```python
from build123d import *

# Parameters (mm, degrees)
F1_DEPTH = 50.8
F2_R     = 25.39999
F4_W     = 61.8233563619
F4_H     = 42.2021473569
F4_W_2   = 44.7444434271
F4_H_2   = 31.3514119965
F5_DEPTH = 50.8


# Not quite as in the source:
# - a fillet or chamfer is up to 0.001 mm smaller than in the source, because OpenCascade refuses the exact size


with BuildPart() as f1:
    # F0 (on Top) → F1 (new body)
    with BuildSketch(Plane.XY):
        with BuildLine():
            Line((-125.9584231198, 326.6096413136), (-125.9584231198, -437.0573322225))
            Line((-125.9584231198, -437.0573322225), (-49.7584231198, -437.0573322225))
            Line((-49.7584231198, -437.0573322225), (77.2415768802, -437.0573322225))
            Line((77.2415768802, -437.0573322225), (77.2415768802, -386.2573322225))
            Line((77.2415768802, -386.2573322225), (-49.7584231198, -386.2573322225))
            Line((-49.7584231198, -386.2573322225), (-49.7584231198, -348.1573322225))
            Line((-49.7584231198, -348.1573322225), (77.2415768802, -348.1573322225))
            Line((77.2415768802, -348.1573322225), (77.2415768802, -297.3573322225))
            Line((77.2415768802, -297.3573322225), (-49.7584231198, -297.3573322225))
            Line((-49.7584231198, -297.3573322225), (-49.7584231198, -259.2573322225))
            Line((-49.7584231198, -259.2573322225), (77.2415768802, -259.2573322225))
            Line((77.2415768802, -259.2573322225), (77.2415768802, -208.4573322225))
            Line((77.2415768802, -208.4573322225), (-49.7584231198, -208.4573322225))
            Line((-49.7584231198, -208.4573322225), (-49.7584231198, 326.6096413136))
            ThreePointArc((-49.7584231198, 326.6096413136), (12.201780711, 376.4463381022), (-23.1943939269, 447.6493859763))
            ThreePointArc((-23.1943939269, 447.6493859763), (-86.3855996742, 517.0444461389), (-149.6523168654, 447.718221991))
            ThreePointArc((-149.6523168654, 447.718221991), (-185.4004633868, 377.8523446501), (-125.9584231198, 326.6096413136))
        make_face()
        with BuildLine():
            ThreePointArc((-86.4201652133, 379.6749489688), (-156.0774751911, 370.9944555466), (-113.7312923812, 426.9792088355))
            ThreePointArc((-113.7312923812, 426.9792088355), (-86.4201652133, 491.6444555466), (-59.1090380455, 426.9792088355))
            ThreePointArc((-59.1090380455, 426.9792088355), (-16.7628552356, 370.9944555466), (-86.4201652133, 379.6749489688))
        make_face(mode=Mode.SUBTRACT)
    extrude(amount=F1_DEPTH)

    # F2 (radius 25.4 in the source; OpenCascade refuses exactly that, so slightly less here)
    f2_edges = [f1.edges().sort_by_distance(p)[0] for p in [
        (-125.958423, -55.223845, 50.8),
        (-49.758423, 59.076155, 50.8),
        (-49.758423, 59.076155, 0),
        (-125.958423, -55.223845, 0),
        (-49.758423, -278.307332, 0),
        (-49.758423, -367.207332, 0),
        (-49.758423, -367.207332, 50.8),
        (-49.758423, -278.307332, 50.8),
    ]]
    fillet(f2_edges, radius=F2_R)

    # F4 (on face) → F5 (cut)
    with BuildSketch(Plane.XY.offset(50.8)):
        with Locations((57.3532550612, -390.556258544)):
            Rectangle(F4_W, F4_H)
        with Locations((74.2137985938, -338.4330382207)):
            Rectangle(F4_W_2, F4_H_2)
    extrude(amount=-F5_DEPTH, mode=Mode.SUBTRACT)


solid = f1.part
```
The model under review builds one solid part; all positions refer to its coordinate system, in mm. A direction names the side the tool comes from. Coordinates: 2 decimals unless noted, no trailing zeros. Write each loop counter-clockwise with the first axis right and the second up, starting at its lowest first coordinate (ties: lowest second). Pieces come first, ordered by that corner, then holes.
1) We need section A-A on x = 1.5. State the section outline as (y, z) points, then the cut area to 3 significant figures.
2) To check wall thickness, follow probe 1 along Y at (x, z) = (53.5, 22.5); probe 2 along Y at (x, z) = (33.5, 41); probe 3 along Y at (x, z) = (-31, 39). State the ranges of each line that lie inside material, in increasing order.
3) Clearance check with flat-ended pins moving along their axes: pin 1 Ø6 at (x, z) = (-19, 29) entering from +Y; pin 2 Ø8 at (x, y) = (-131, -11) entering from +Z; pin 3 Ø20.5 at (y, z) = (-396.5, 34.5) entering from +X; pin 4 Ø4 at (x, z) = (-77, 33.5) entering from +Y. State where each tip first meets the part, or that it passes through.
4) We need section B-B on z = 9. State the section outline as (x, y) points, then the cut area to 3 significant figures.
5) The part is to be moulded in two halves that separate along X. For faces 1 (the face through (19, -297.357, 25)), 2 (the face through (-16.156, 372.087, 25.044)), 3 (the face through (51.842, -336, 26)), say which applies: pulls with the +X half, pulls with the -X half, needs draft (parallel to the pull), parting line crosses it, or undercut.
6) Machinability: for faces 4 (the face through (64, -322.757, 26)), 5 (the face through (-57, -366.94, 43.16)), 6 (the face through (-57, -366.94, 7.64)), 7 (the face through (77.242, -310, 25)), which of the approach directions +Z, -Z, +X, -X, +Y, -Y give a long, thin tool a straight path to every point of the face, cutting with its end or side? Answer none if there is none.
Answer list:
1. outline: (-437.06, 0) - (-386.26, 0) - (-386.26, 50.8) - (-437.06, 50.8) - close; (-348.16, 0) - (-297.36, 0) - (-297.36, 50.8) - (-348.16, 50.8) - close; (-259.26, 0) - (-208.46, 0) - (-208.46, 50.8) - (-259.26, 50.8) - close; (352.67, 0) - (427.41, 0) - (427.41, 50.8) - (352.67, 50.8) - close
1. area: 11,500 mm2
2. probe 1: y = -437.06 to -411.66, -322.76 to -297.36, -259.26 to -208.46
2. probe 2: y = -437.06 to -411.66, -348.16 to -297.36, -259.26 to -208.46
2. probe 3: y = -437.06 to -386.26, -348.16 to -297.36, -259.26 to -208.46, 329.45 to 356.88, 423.21 to 484.54
3. pin 1: stops at y = 447.08
3. pin 2: passes through
3. pin 3: stops at x = 26.44
3. pin 4: stops at y = 516.61
4. outline: (-149.65, 447.72) arc R63.5 ccw to (-119.95, 326.62) - (-119.95, -437.06) - (77.24, -437.06) - (77.24, -411.66) - (26.44, -411.66) - (26.44, -386.26) - (-55.76, -386.26) - (-55.76, -348.16) - (51.84, -348.16) - (51.84, -322.76) - (77.24, -322.76) - (77.24, -297.36) - (-55.76, -297.36) - (-55.76, -259.26) - (77.24, -259.26) - (77.24, -208.46) - (-55.76, -208.46) - (-55.76, 326.89) arc R63.43 ccw to (-23.19, 447.65) arc R63.5 ccw (long way) to start; hole (-113.73, 426.98) arc R38.1 ccw (long way) to (-86.42, 379.67) arc R38.1 ccw (long way) to (-59.11, 426.98) arc R38.1 ccw (long way) to start
4. area: 82,100 mm2
5. face 1: needs draft
5. face 2: undercut
5. face 3: pulls with the +X half
6. face 4: +Z, -Z, +X
6. face 5: +Z, +X
6. face 6: -Z, +X
6. face 7: +Z, -Z, +X, +Y, -Y
